Geometry: final body of the model. Coordinates: model frame, mm. A direction names the side the tool comes from. Give positions to 0.01 mm unless a question says otherwise; leave off trailing zeros. Write each loop counter-clockwise with the first axis right and the second up, starting at its lowest first coordinate (ties: lowest second). Pieces come first, ordered by that corner, then holes. Notation, with made-up numbers: (-11, 51.5) -> (41, 51.5) arc R24 ccw to (41, 77.5) -> close; hole circle Ø3 at (2.5, 83.5). An arc over 180 degrees is marked (long way). Answer as a JSON object with one key per item and string values.
from build123d import *

# Parameters (mm, degrees)
F0_W      = 25
F0_H      = 25
F1_DEPTH  = 2
F2_R      = 1.65
F6_DEPTH  = 3
F3_R      = 1.65
F7_DEPTH  = 3
F4_R      = 1.65
F8_DEPTH  = 3
F5_R      = 1.65
F9_DEPTH  = 3
F10_R     = 3.5
F11_W     = 2
F11_H     = 7
F12_DEPTH = 23
F14_W     = 7
F14_H     = 12
F15_DEPTH = 3
F16_W     = 7
F16_H     = 3.2
F17_DEPTH = 3
F19_R     = 1.025
F20_DEPTH = 6
F18_R     = 1.025
F21_DEPTH = 6
F13_R     = 1
F22_DEPTH = 3
F23_SIZE  = 1
F24_DEPTH = 1
F25_DEPTH = 1


with BuildPart() as f1:
    # F0 (on Top) → F1 (new body)
    with BuildSketch(Plane.XY):
        with Locations((12.5, 12.5)):
            Rectangle(F0_W, F0_H)
    extrude(amount=F1_DEPTH)

    # F2 (on face) → F6 (cut)
    with BuildSketch(Plane.XY.offset(2)):
        with Locations((3.5, 21.5)):
            Circle(F2_R)
    extrude(amount=-F6_DEPTH, mode=Mode.SUBTRACT)

    # F3 (on face) → F7 (cut)
    with BuildSketch(Plane.XY.offset(2)):
        with Locations((21.5, 21.5)):
            Circle(F3_R)
    extrude(amount=-F7_DEPTH, mode=Mode.SUBTRACT)

    # F4 (on face) → F8 (cut)
    with BuildSketch(Plane.XY.offset(2)):
        with Locations((3.5, 3.5)):
            Circle(F4_R)
    extrude(amount=-F8_DEPTH, mode=Mode.SUBTRACT)

    # F5 (on face) → F9 (cut)
    with BuildSketch(Plane.XY.offset(2)):
        with Locations((21.5, 3.5)):
            Circle(F5_R)
    extrude(amount=-F9_DEPTH, mode=Mode.SUBTRACT)

    # F10
    f10_edges = [f1.edges().sort_by_distance(p)[0] for p in [
        (0, 0, 1),
        (0, 25, 1),
        (25, 25, 1),
        (25, 0, 1),
    ]]
    fillet(f10_edges, radius=F10_R)

    # F11 (on face) → F12 (join)
    with BuildSketch(Plane.XY.offset(2)):
        with Locations((10, 12.5)):
            Rectangle(F11_W, F11_H)
    extrude(amount=F12_DEPTH)

    # F14 (on face) → F15 (join)
    with BuildSketch(Plane.YZ.offset(11)):
        with Locations((12.5, 19)):
            Rectangle(F14_W, F14_H)
    extrude(amount=F15_DEPTH)

    # F16 (on face) → F17 (cut)
    with BuildSketch(Plane.YZ.offset(14)):
        with Locations((12.5, 19)):
            Rectangle(F16_W, F16_H)
    extrude(amount=-F17_DEPTH, mode=Mode.SUBTRACT)

    # F19 (on face) → F20 (cut)
    with BuildSketch(Plane.YZ.offset(14)):
        with Locations((12.5, 15.2)):
            Circle(F19_R)
    extrude(amount=-F20_DEPTH, mode=Mode.SUBTRACT)

    # F18 (on face) → F21 (cut)
    with BuildSketch(Plane.YZ.offset(14)):
        with Locations((12.5, 22.8)):
            Circle(F18_R)
    extrude(amount=-F21_DEPTH, mode=Mode.SUBTRACT)

    # F13 (on face) → F22 (cut)
    with BuildSketch(Plane.YZ.offset(11)):
        with Locations((12.5, 19.1)):
            Circle(F13_R)
    extrude(amount=-F22_DEPTH, mode=Mode.SUBTRACT)

    # F23
    f23_edges = [f1.edges().sort_by_distance(p)[0] for p in [
        (9, 11.5, 19.1),
    ]]
    chamfer(f23_edges, length=F23_SIZE)

    # F24 (add): a face of the model
    f24_faces = [f1.faces().sort_by_distance(p)[0] for p in [
        (11.5, 12.5, 25),
    ]]
    extrude(f24_faces, amount=F24_DEPTH)

    # F25 (add): a face of the model
    f25_faces = [f1.faces().sort_by_distance(p)[0] for p in [
        (12.5, 12.5, 13),
    ]]
    extrude(f25_faces, amount=F25_DEPTH)


solid = f1.part
Q1. Mould query, pull axis Y, two halves, no side actions, for faces 1 (the flat face through (14, 12, 24)), 2 (the cylindrical face through (1, 1.05, 1.01)), 3 (the cylindrical face through (1.85, 3.57, 1.01)). Classes: pulls with the +Y half, pulls with the -Y half, needs draft (parallel to the pull), parting line crosses it, or undercut.
Values:
{"face 1": "needs draft", "face 2": "pulls with the -Y half", "face 3": "undercut"}
Q2. Cut plane A-A (x = 13). Return the cut outline in (y, z) (3 decimals).
Values:
{"outline": "(0, 0) -> (25, 0) -> (25, 2) -> (0, 2) -> close; (9, 12) -> (16, 12) -> (16, 17.4) -> (9, 17.4) -> close; (9, 20.6) -> (16, 20.6) -> (16, 26) -> (9, 26) -> close; hole circle Ø2.05 at (12.5, 15.2); hole circle Ø2.05 at (12.5, 22.8)"}
Q3. Cut plane C-C (y = 8). Return the cut outline in (x, z), and give its area (3 significant figures).
Values:
{"outline": "(0, 0) -> (25, 0) -> (25, 2) -> (0, 2) -> close", "area": "50.0 mm²"}
Q4. Set-up query: faces 4 (the flat face through (9, 12, 14)), 5 (the flat face through (13, 12, 20.6)), 6 (the flat face through (11, 16, 17)). Return all of +Z, -Z, +X, -X, +Y, -Y with unobstructed straight access to the full face (end or side cutting, diameter ignored); none if empty.
Values:
{"face 4": "+Z, -X, +Y, -Y", "face 5": "+X, +Y, -Y", "face 6": "+Z, +X, -X, +Y"}
Q5. First-contact query: P1, Ø2.5, axis at x = 3.5, y = 21.5, coming from the +Z side; P2, Ø5.5, axis at x = 10.5, z = 13, coming from the +Y side; P3, Ø7.5, axis at y = 14, z = 12, coming from the -X side; P4, Ø5, axis at y = 12.5, z = 14, coming from the +X side. Flat tips, straight axial feed; report the tip coordinate or a pass-through.
Values:
{"P1": "through", "P2": "y = 16", "P3": "x = 9", "P4": "x = 14"}
Q6. Material intervals for L1, parallel to Y at x = 3.5, z = 0.9; L2, parallel to Z at x = 10.7, y = 12.5 (3 decimals); L3, parallel to Y at x = 9.25, z = 2.75, sorted ascending. Write a range as from..to.
Values:
{"L1": "0..1.85, 5.15..19.85, 23.15..25", "L2": "0..14.175, 16.225..18.1, 20.1..21.775, 23.825..26", "L3": "9..16"}
Q7. Cut plane B-B (z = 15.2). Return the cut outline in (x, y) (3 decimals).
Values:
{"outline": "(9, 9) -> (14, 9) -> (14, 11.475) -> (9, 11.475) -> close; (9, 13.525) -> (14, 13.525) -> (14, 16) -> (9, 16) -> close"}
Q8. Cut plane D-D (x = 2.5). Return the cut outline in (y, z), and give its area (3 significant figures).
Values:
{"outline": "(0.15, 0) -> (2.19, 0) -> (2.19, 2) -> (0.15, 2) -> close; (4.81, 0) -> (20.19, 0) -> (20.19, 2) -> (4.81, 2) -> close; (22.81, 0) -> (24.85, 0) -> (24.85, 2) -> (22.81, 2) -> close", "area": "38.9 mm²"}
